For this review, take the finished solid that the model builds, in its own axes (mm). A direction names the side the tool comes from. Give positions to 0.01 mm unless a question says otherwise; leave off trailing zeros. Order: outer loops, then holes, each group sorted by start corner. A loop starts at its lowest first (then second) coordinate and runs counter-clockwise, first axis right, second up.
Item 1: For P1, Ø8, axis at x = 0.43, z = 5.25, coming from the -Y side; P2, Ø2, axis at y = -11, z = -2.5, coming from the -X side; P3, Ø2, axis at x = 0, z = 3.5, coming from the -Y side; P4, Ø1.5, axis at x = 13, y = -6, coming from the -Z side, all flat-tipped, find the tip position at first contact; note any pin that passes through.
Item 2: Consider section D-D (y = -7). Give the boundary of the cut face in (x, z), plus the area to 3 significant figures.
Item 3: Machinability: for faces 4 (the flat face through (9, -18, 0)), 5 (the flat face through (6.521, -13, -3)), 6 (the flat face through (2.5, -7.753, 2.5)), 7 (the flat face through (14, -6, 0)), which of the approach directions +Z, -Z, +X, -X, +Y, -Y give a long, thin tool a straight path to every point of the face, cutting with its end or side? Answer none if there is none.
Item 4: Consider section A-A (z = 7). Give the boundary of the cut face in (x, y), plus the area to 3 significant figures.
Item 5: For probe 1 along X at (y, z) = (-9.35, 5.25); probe 2 along X at (y, z) = (-5.5, 5.25); probe 3 along X at (y, z) = (-7.25, 8.5), list the stretches that pass through material, from the lowest coordinate up.
Item 6: Consider section B-B (y = -12). Give the boundary of the cut face in (x, z).
Item 7: The part is to be moulded in two halves that separate along Z. For faces 1 (the cylindrical face through (8.794, -5.766, 2.153)), 2 (the flat face through (8, -25.203, -2)), 3 (the flat face through (0, -6, 9.3)), say which applies: released by +Z, released by -Z, zero draft, split by the parting line, or undercut.
Item 8: Consider section C-C (z = -2.5). Give the boundary of the cut face in (x, y).
Autodesk Inventor part; units mm, degrees
ref_plane "YZ Plane" through (0, 0, 0) normal (1, 0, 0) x (0, 1, 0)
ref_plane "XZ Plane" through (0, 0, 0) normal (0, 1, 0) x (-1, 0, 0)
ref_plane "XY Plane" through (0, 0, 0) normal (0, 0, 1) x (1, 0, 0)
sketch "Skizze1" plane through (0, 0, 0) normal (0, 0, 1) x (1, 0, 0)
  point P0 (0, 0)
sketch "Skizze2" plane through (0, 0, 0) normal (0, 0, 1) x (1, 0, 0)
  line L0 (-15.5739, -1.2028) -> (16.4261, -1.2028)
  line L1 (16.4261, -1.2028) -> (16.4261, -10.2028)
  line L2 (16.4261, -10.2028) -> (-15.5739, -10.2028)
  line L3 (-15.5739, -10.2028) -> (-15.5739, -1.2028)
  point P0 (0, 0)
  dimension "d0" = 32
  dimension "d1" = 9
extrude "Extrusion1" add sketch "Skizze2" along normal blind 10.5
sketch "Skizze3" plane through (16.4261, -10.2028, 0) normal (1, 0, 0) x (0, 0, -1)
  point P0 (0, 10.2028)
sketch "Skizze4" plane through (-15.5739, -1.2028, 0) normal (0, 1, 0) x (1, 0, 0)
  line L0 (0, 0) -> (0, -10.5)
  line L1 (0, 0) -> (32, 0)
  point P0 (15.5739, 0)
  point P1 (16, -5.25)
  point P2 (7.496, -5.25)
  point P3 (24.504, -5.25)
  dimension "d4" = 8.504
  dimension "d5" = 8.504
  dimension "d6" = 16
  dimension "d14" = 5.25
  dimension "d15" = 5.25
sketch "Skizze5" plane through (0, 0, 0) normal (0, 0, -1) x (-1, 0, 0)
  point P0 (0, 0)
sketch "Skizze6" plane through (0, 0, 0) normal (0, 0, -1) x (-1, 0, 0)
  line L0 (-4.8511, -7.7528) -> (3.9989, -7.7528)
  line L1 (3.9989, -7.7528) -> (3.9989, -3.6528)
  line L2 (3.9989, -3.6528) -> (-4.8511, -3.6528)
  line L3 (-4.8511, -3.6528) -> (-4.8511, -7.7528)
  line L4 (-16.4261, -10.2028) -> (15.5739, -10.2028)
  line L5 (15.5739, -10.2028) -> (15.5739, -1.2028)
  point P0 (0, 0)
  dimension "d16" = 8.85
  dimension "d17" = 4.1
  dimension "d18" = 2.45
  dimension "d19" = 11.575
extrude "Extrusion2" cut sketch "Skizze6" against normal blind 9.3
sketch "Skizze7" plane through (-15.5739, -10.2028, 0) normal (0, -1, 0) x (1, 0, 0)
  point P0 (15.5739, 0)
sketch "Skizze8" plane through (0, 0, 0) normal (0, 0, -1) x (-1, 0, 0)
  point P0 (0, 0)
sketch "Skizze9" plane through (-15.5739, -10.2028, 0) normal (0, -1, 0) x (1, 0, 0)
  line L0 (0, 0) -> (32, 0)
  line L1 (4.9045, 0) -> (9.9045, 0)
  line L2 (9.9045, 0) -> (9.9045, 1.2)
  line L3 (9.9045, 1.2) -> (4.9045, 1.2)
  line L4 (4.9045, 1.2) -> (4.9045, 0)
  point P0 (15.5739, 0)
  dimension "d22" = 1.2
  dimension "d23" = 5
extrude "Extrusion3" add sketch "Skizze9" along normal blind 15
sketch "Skizze10" plane through (0, 0, 0) normal (0, 0, -1) x (-1, 0, 0)
  line L0 (5.6694, -25.2028) -> (10.6694, -25.2028)
  line L1 (15.5739, -1.2028) -> (-16.4261, -1.2028)
  line L2 (10.6694, -25.2028) -> (5.6694, -25.2028)
  line L3 (5.6694, -25.2028) -> (5.6694, -1.2028)
  line L4 (5.6694, -1.2028) -> (10.6694, -1.2028)
  line L5 (10.6694, -1.2028) -> (10.6694, -25.2028)
  point P0 (0, 0)
  dimension "d26" = 5
extrude "Extrusion4" add sketch "Skizze10" along normal blind 5
sketch "Skizze11" plane through (-15.5739, -25.2028, 0) normal (0, -1, 0) x (1, 0, 0)
  line L0 (4.9045, -5) -> (9.9045, -5)
  line L1 (6.7795, -5) -> (8.0295, -5)
  line L2 (8.0295, -5) -> (8.0295, -0.9525)
  line L3 (8.0295, -0.9525) -> (6.7795, -0.9525)
  line L4 (6.7795, -0.9525) -> (6.7795, -5)
  line L5 (9.9045, 1.2) -> (9.9045, -5)
  point P0 (15.5739, 0)
  dimension "d29" = 1.25
  dimension "d30" = 1.875
  dimension "d31" = 4.0475
extrude "Extrusion5" cut sketch "Skizze11" against normal blind 22
sketch "Skizze12" plane through (-15.5739, -25.2028, 0) normal (0, -1, 0) x (1, 0, 0)
  line L0 (9.9045, 1.2) -> (9.9045, 0)
  line L1 (4.9045, 0) -> (4.9045, 1.2)
  line L2 (9.9045, 1.2) -> (4.9045, 1.2)
  line L3 (4.9045, 1.2) -> (4.9045, 0)
  line L4 (4.9045, 0) -> (9.9045, 0)
  line L5 (9.9045, 0) -> (9.9045, 1.2)
  point P0 (15.5739, 0)
extrude "Extrusion6" cut sketch "Skizze12" against normal blind 15
sketch "Skizze13" plane through (0, 0, 0) normal (0, 1, 0) x (-1, 0, 0)
  line L0 (5.6694, 0) -> (-16.4261, 0)
  line L1 (-6.5211, 0) -> (-11.5211, 0)
  line L2 (-11.5211, 0) -> (-11.5211, -5)
  line L3 (-11.5211, -5) -> (-6.5211, -5)
  line L4 (-6.5211, -5) -> (-6.5211, 0)
  line L5 (-16.4261, 0) -> (-16.4261, 10.5)
  point P0 (0, 0)
  dimension "d36" = 5
  dimension "d37" = 5
  dimension "d38" = 4.905
extrude "Extrusion7" add sketch "Skizze13" against normal blind 25.203
sketch "Skizze14" plane through (6.5211, 0, 0) normal (0, 0, 1) x (1, 0, 0)
  line L0 (5, -1.2028) -> (9.905, -1.2028)
  line L1 (0, 0) -> (0, -25.203)
  line L2 (5, -1.2028) -> (0, -1.2028)
  line L3 (0, -1.2028) -> (0, 0)
  line L4 (0, 0) -> (5, 0)
  line L5 (5, 0) -> (5, -1.2028)
  point P0 (-6.5211, 0)
extrude "Extrusion8" cut sketch "Skizze14" against normal blind 25
sketch "Skizze15" plane through (0, -25.203, 0) normal (0, -1, 0) x (1, 0, 0)
  line L0 (6.5211, -5) -> (11.5211, -5)
  line L1 (8.3961, -5) -> (9.6461, -5)
  line L2 (9.6461, -5) -> (9.6461, -0.952)
  line L3 (9.6461, -0.952) -> (8.3961, -0.952)
  line L4 (8.3961, -0.952) -> (8.3961, -5)
  line L5 (11.5211, -5) -> (11.5211, 0)
  point P0 (0, 0)
  dimension "d43" = 1.25
  dimension "d44" = 4.048
  dimension "d45" = 1.875
extrude "Extrusion9" cut sketch "Skizze15" against normal blind 22
sketch "Skizze16" plane through (-15.5739, -25.2028, 0) normal (0, -1, 0) x (1, 0, 0)
  line L0 (0, 0) -> (4.9045, 0)
  line L1 (4.9045, -5) -> (9.9045, -5)
  line L2 (4.9045, 0) -> (9.9045, 0)
  line L3 (9.9045, 0) -> (9.9045, -5)
  line L4 (9.9045, -5) -> (4.9045, -5)
  line L5 (4.9045, -5) -> (4.9045, 0)
  point P0 (15.5739, 0)
extrude "Extrusion10" cut sketch "Skizze16" against normal blind 25
hole "Bohrung2" at (0.4261, -1.2028, 5.25) direction (0, -1, 0) diameter 6 end through all
hole "Bohrung3" at (-8.0779, -1.2028, 5.25) at (8.9301, -1.2028, 5.25) direction (0, -1, 0) diameter 6.2 end through all
properties part number "Objektträgerhalter 3a Neu"
Resolved:
1. P1: stops at y = -10.2
1. P2: stops at x = 6.52
1. P3: passes through
1. P4: stops at z = 0
2. outline: (-15.57, 0) - (-4, 0) - (-4, 9.3) - (4.85, 9.3) - (4.85, 0) - (6.52, 0) - (6.52, -5) - (8.4, -5) - (8.4, -0.95) - (9.65, -0.95) - (9.65, -5) - (11.52, -5) - (11.52, 0) - (16.43, 0) - (16.43, 10.5) - (-15.57, 10.5) - close; hole circle Ø6.2 at (-8.08, 5.25); hole circle Ø6.2 at (8.93, 5.25)
2. area: 213 mm2
3. face 4: +Z, +X, -X, -Y
3. face 5: -Z, -X, +Y, -Y
3. face 6: -Z
3. face 7: -Z, +X, +Y, -Y
4. outline: (-15.57, -10.2) - (-10.64, -10.2) - (-10.64, -1.2) - (-15.57, -1.2) - close; (-5.52, -10.2) - (-2.01, -10.2) - (-2.01, -7.75) - (-4, -7.75) - (-4, -3.65) - (-2.01, -3.65) - (-2.01, -1.2) - (-5.52, -1.2) - close; (2.86, -10.2) - (6.37, -10.2) - (6.37, -1.2) - (2.86, -1.2) - (2.86, -3.65) - (4.85, -3.65) - (4.85, -7.75) - (2.86, -7.75) - close; (11.49, -10.2) - (16.43, -10.2) - (16.43, -1.2) - (11.49, -1.2) - close
4. area: 136 mm2
5. probe 1: x = -15.57 to -11.18, -4.98 to -2.57, 3.43 to 5.83, 12.03 to 16.43
5. probe 2: x = -15.57 to -11.18, -4.98 to -4, 4.85 to 5.83, 12.03 to 16.43
5. probe 3: x = -15.57 to -4, 4.85 to 16.43
6. outline: (6.52, -5) - (8.4, -5) - (8.4, -0.95) - (9.65, -0.95) - (9.65, -5) - (11.52, -5) - (11.52, 0) - (6.52, 0) - close
7. face 1: undercut
7. face 2: zero draft
7. face 3: released by -Z
8. outline: (6.52, -25.2) - (8.4, -25.2) - (8.4, -3.2) - (9.65, -3.2) - (9.65, -25.2) - (11.52, -25.2) - (11.52, -1.2) - (6.52, -1.2) - close
